```python
from build123d import *

# Parameters (mm, degrees)
F0_W     = 138
F0_H     = 70
F1_DEPTH = 7
F2_R     = 11.346804
F3_R     = 3
F4_W     = 26.570709
F4_H     = 2.072412
F5_DEPTH = 0.5
F6_W     = 13.949622
F6_H     = 2.113027
F7_DEPTH = 0.5


with BuildPart() as f1:
    # F0 (on Top) → F1 (new body)
    with BuildSketch(Plane.XY):
        Rectangle(F0_W, F0_H)
    extrude(amount=F1_DEPTH)

    # F2
    f2_edges = [f1.edges().sort_by_distance(p)[0] for p in [
        (69, -35, 3.5),
        (69, 35, 3.5),
        (-69, -35, 3.5),
        (-69, 35, 3.5),
    ]]
    fillet(f2_edges, radius=F2_R)

    # F3
    f3_edges = [f1.edges().sort_by_distance(p)[0] for p in [
        (0, 35, 0),
        (0, -35, 0),
        (-69, 0, 0),
        (69, 0, 0),
    ]]
    fillet(f3_edges, radius=F3_R)

    # F4 (on face) → F5 (join)
    with BuildSketch(Plane.XZ.offset(35)):
        with Locations((-40.915458, 4.036206)):
            Rectangle(F4_W, F4_H)
    extrude(amount=F5_DEPTH)

    # F6 (on face) → F7 (join)
    with BuildSketch(Plane(origin=(0, 35, 0), x_dir=(-1, 0, 0), z_dir=(0, 1, 0))):
        with Locations((29.512195, 4.056513)):
            Rectangle(F6_W, F6_H)
    extrude(amount=F7_DEPTH)


solid = f1.part
```
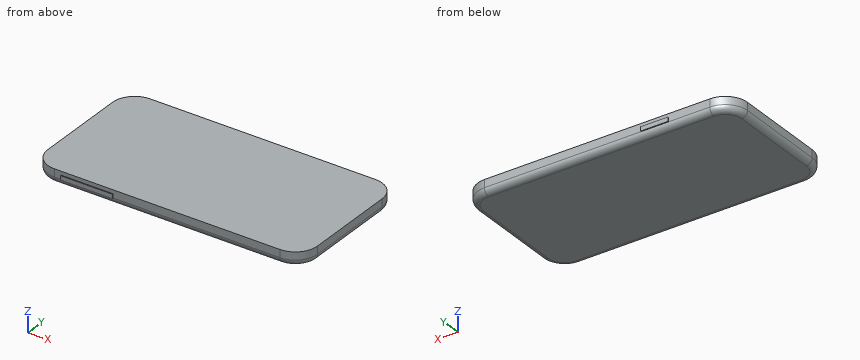
CAD build for the part. Positions are in the model's coordinates, mm. Coordinates: 2 decimals unless noted, no trailing zeros. Write each loop counter-clockwise with the first axis right and the second up, starting at its lowest first coordinate (ties: lowest second). Pieces come first, ordered by that corner, then holes. Notation, with made-up numbers: (0, -21) -> (32, -21) arc R8 ccw to (32, -17) -> close; hole circle Ø10 at (76, 41). An arc over 180 degrees is marked (long way). Return JSON: item names as keys, results as strings. Group by question number.
Q1. Cut at A-A, the plane x = -17. Give the cut face in (y, z).
Q2. Flat gauge pins, fed straight in: pin 1 (2 mm diameter, centred on x = 8.5, z = 5, fed in from +Y); pin 2 (0.6 mm diameter, centred on y = 35.5, z = 4.5, fed in from -X); pin 3 (2 mm diameter, centred on x = 9, z = 4.5, fed in from -Y). Where does each tip first touch, or does it go through?
Q3. Cut at B-B, the plane z = 1.5. Give the cut face in (x, y), then the cut area to 3 significant figures.
Q4. Drill centre lines: line 1 (Y direction, x = -42, z = 3.5); line 2 (Y direction, x = 25.5, z = 3.5); line 3 (X direction, y = 16, z = 1.5). Where is each one in solid material? Low to high.
Q5. Cut at C-C, the plane x = -51.5. Give the cut face in (y, z).
Returned:
{
 "1": {"outline": "(-35, 3) arc R3 ccw to (-32, 0) -> (32, 0) arc R3 ccw to (35, 3) -> (35, 7) -> (-35, 7) -> close"},
 "2": {"pin 1": "stops at y = 35", "pin 2": "stops at x = -36.49", "pin 3": "stops at y = -35"},
 "3": {"outline": "(-68.6, -23.65) arc R10.94 ccw to (-57.65, -34.6) -> (57.65, -34.6) arc R10.94 ccw to (68.6, -23.65) -> (68.6, 23.65) arc R10.94 ccw to (57.65, 34.6) -> (-57.65, 34.6) arc R10.94 ccw to (-68.6, 23.65) -> close", "area": "9,390 mm2"},
 "4": {"line 1": "y = -35.5 to 35", "line 2": "y = -35 to 35", "line 3": "x = -68.6 to 68.6"},
 "5": {"outline": "(-35.5, 3) -> (-35, 3) arc R3 ccw to (-32, 0) -> (32, 0) arc R3 ccw to (35, 3) -> (35, 7) -> (-35, 7) -> (-35, 5.07) -> (-35.5, 5.07) -> close"}
}
